Input: part model. Units: mm. Frame: model coordinates. A direction names the side the tool comes from. Give positions to 0.01 mm unless a question says otherwise; leave off trailing zeros. Loops run counter-clockwise (first coordinate to the right, second up) from the corner with the lowest first, then second, coordinate; pieces in that order, holes last. Notation, with made-up numbers: (-26.5, 87) - (-19.5, 87) arc R21 ccw to (-19.5, 109) - close; hole circle Ø7 at (-29, 21). An arc over 180 degrees is marked (long way). Answer as a JSON object with one key per item and string values. Group by question number.
(1) Section query B-B (y = -32). Return loops of the section in (x, z), plus the area to 3 significant figures.
(2) Access query for faces 4 (the flat face through (-9, -20, 1)), 5 (the flat face through (-5.833, 1, 1)), 6 (the flat face through (-13.5, 2, 1)), 7 (the flat face through (3, -29.167, 1)), 8 (the flat face through (0, -15, 1)). Directions: +Z, -Z, +X, -X, +Y, -Y. A direction counts if a zero-diameter tool reaches every point of the face in a straight line with its end or side. Return the directions, or none.
(3) Material intervals for L1, parallel to Y at x = 3, z = 2; L2, parallel to Y at x = -30, z = 1.65, sorted ascending.
(4) Section query A-A (x = 0.5). Return loops of the section in (y, z).
(5) Pin query (flat end, axial travel): P1, Ø1.5, axis at y = 2, z = 1, coming from the +X side; P2, Ø0.9, axis at x = 4, z = 1, coming from the -Y side; P3, Ø0.6, axis at y = -1.5, z = 1.5, coming from the -X side. Return the tip coordinate at first contact, or that it passes through.
(6) Mould query, pull axis Y, two halves, no side actions, for faces 1 (the flat face through (0, -32, 1)), 2 (the flat face through (-18, -5, 1)), 3 (the flat face through (-15, -4.5, 1)). Classes: +Y half, -Y half, draft (parallel to the pull), parting line (faces both ways), or undercut.
(7) Section query C-C (x = -27). Return loops of the section in (y, z).
Autodesk Inventor part; units mm, degrees
ref_plane "YZ Plane" through (0, 0, 0) normal (1, 0, 0) x (0, 1, 0)
ref_plane "XZ Plane" through (0, 0, 0) normal (0, 1, 0) x (-1, 0, 0)
ref_plane "XY Plane" through (0, 0, 0) normal (0, 0, 1) x (1, 0, 0)
sketch "Sketch2" plane through (0, 0, 0) normal (0, 0, 1) x (1, 0, 0)
  line L0 (0, 0) -> (0, -5.8333)
  line L1 (0, -35) -> (-35, 0)
  line L2 (-35, 0) -> (-29.1667, 0)
  line L3 (-5.8333, 0) -> (-5.8333, 3)
  line L4 (-5.8333, 3) -> (-13.5, 3)
  line L5 (-13.5, 3) -> (-13.5, 0)
  line L6 (-21.5, 0) -> (-21.5, 3)
  line L7 (-21.5, 3) -> (-29.1667, 3)
  line L8 (-29.1667, 3) -> (-29.1667, 0)
  line L9 (-17.5, 7.0256) -> (-17.5, -7.5618) construction
  line L10 (-19, 0) -> (-19, -2)
  line L11 (-19, -2) -> (-20.2, -2)
  line L12 (-20.2, -2) -> (-20.2, -4.5)
  line L13 (-20.2, -4.5) -> (-19, -4.5)
  line L14 (-19, -4.5) -> (-19, -5)
  line L15 (-19, -5) -> (-16, -5)
  line L16 (-16, -5) -> (-16, -4.5)
  line L17 (-16, -4.5) -> (-14.8, -4.5)
  line L18 (-14.8, -4.5) -> (-14.8, -2)
  line L19 (-14.8, -2) -> (-16, -2)
  line L20 (-16, 0) -> (-16, -2)
  line L21 (-16, 0) -> (-13.5, 0)
  line L22 (-21.5, 0) -> (-19, 0)
  line L23 (-5.8333, 0) -> (0, 0)
  line L24 (0, -5.8333) -> (6, -5.8333)
  line L25 (6, -5.8333) -> (6, -13.5)
  line L26 (6, -13.5) -> (0, -13.5)
  line L27 (0, -21.5) -> (6, -21.5)
  line L28 (6, -21.5) -> (6, -29.1667)
  line L29 (6, -29.1667) -> (0, -29.1667)
  line L30 (0, -16) -> (-6.5, -16)
  line L31 (-9, -16) -> (-10, -16)
  line L32 (-10, -16) -> (-10, -19)
  line L33 (-10, -19) -> (-9, -19)
  line L34 (-9, -19) -> (-9, -20.2)
  line L35 (-9, -20.2) -> (-6.5, -20.2)
  line L36 (-6.5, -20.2) -> (-6.5, -19)
  line L37 (-6.5, -19) -> (0, -19)
  line L38 (-12.8614, -17.5) -> (7.6104, -17.5) construction
  line L39 (-9, -16) -> (-9, -14.8)
  line L40 (-9, -14.8) -> (-6.5, -14.8)
  line L41 (-6.5, -14.8) -> (-6.5, -16)
  line L42 (0, -13.5) -> (0, -16)
  line L43 (0, -19) -> (0, -21.5)
  line L44 (0, -29.1667) -> (0, -35)
  dimension "d2" = 35
  dimension "d5" = 3
  dimension "d6" = 3
  dimension "d7" = 5
  dimension "d8" = 8
  dimension "d9" = 2.5
  dimension "d10" = 5.4
  dimension "d11" = 8
  dimension "d12" = 23.3333
  dimension "d13" = 35
  dimension "d14" = 6
  dimension "d15" = 3
  dimension "d17" = 16
  dimension "d18" = 2.5
  dimension "d19" = 5.4
  dimension "d20" = 1
  dimension "d21" = 8
  dimension "d22" = 23.3333
extrude "Extrusion1" add sketch "Sketch2" along normal blind 3
equation "\"d12\" = 0.666667 * d2"
equation "\"d13\" = d2"
equation "\"d22\" = 0.666667 * d13"
properties part number "angle"
Recorded:
{
 "1": {"outline": "(-3, 0) - (0, 0) - (0, 3) - (-3, 3) - close", "area": "9.00 mm^2"},
 "2": {"face 4": "+Z, -Z", "face 5": "+Z, -Z, +X, +Y", "face 6": "+Z, -Z, +Y", "face 7": "+Z, -Z, +X, -Y", "face 8": "+Z, -Z, +X"},
 "3": {"L1": "y = -29.17 to -21.5, -13.5 to -5.83", "L2": "y = -5 to 0"},
 "4": {"outline": "(-29.17, 0) - (-21.5, 0) - (-21.5, 3) - (-29.17, 3) - close; (-13.5, 0) - (-5.83, 0) - (-5.83, 3) - (-13.5, 3) - close"},
 "5": {"P1": "stops at x = -5.83", "P2": "stops at y = -29.17", "P3": "stops at x = -33.8"},
 "6": {"face 1": "draft", "face 2": "+Y half", "face 3": "undercut"},
 "7": {"outline": "(-8, 0) - (3, 0) - (3, 3) - (-8, 3) - close"}
}
